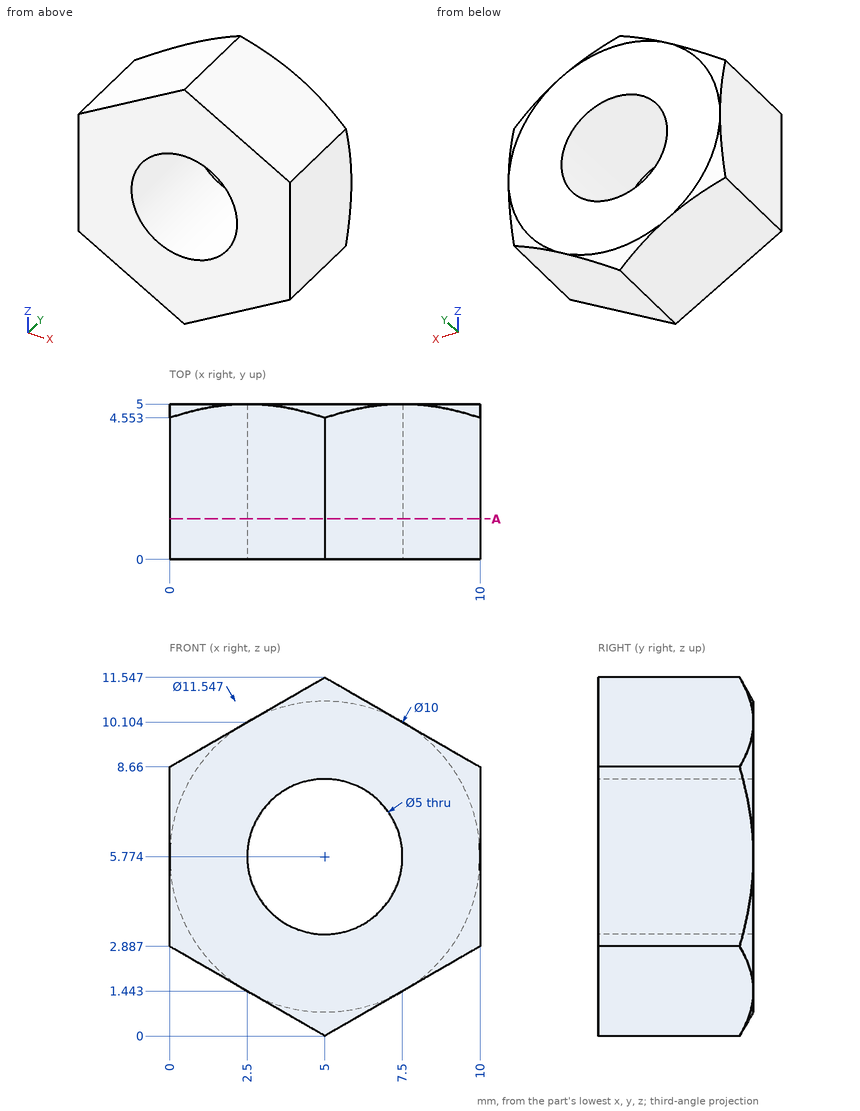
Study the drawing (mm; zero at the part's minimum x, y, z) and answer. Give positions to 0.01 mm unless a question says otherwise; leave off trailing zeros. Write each loop counter-clockwise with the first axis right and the second up, starting at its lowest first coordinate (ties: lowest second). Pieces come first, ordered by that corner, then holes. Notation, with made-up numbers: (-10.75, -27) - (37.25, -27) arc R22 ccw to (37.25, -9) - close; hole circle Ø10 at (52, 61.5). An arc over 180 degrees is marked (long way). One line per question, with ' | ' between items. Start each with the question number.
1. Straight lines are drawn through the part: line 1 (X direction, y = 2.4, z = 5.5) (1 decimal); line 2 (X direction, y = 3.55, z = 8) (1 decimal); line 3 (Z direction, x = 7, y = 4.05) (1 decimal). For each, find the intervals that lie inside material, in ascending order.
2. Given P1, Ø1, axis at y = 1.5, z = 1.5, coming from the +X side (1 decimal); P2, Ø1.5, axis at x = 1.5, y = 3, coming from the -Z side; P3, Ø2, axis at x = 7.5, y = 4, coming from the +Z side, each flat-ended and moving along its own axis, determine where each tip first touches the part or whether it passes through.
3. Section A-A, the plane y = 1.3 is taken. Determine the outline of the cut face in (x, z).
Result:
1) line 1: x = 0 to 2.5, 7.5 to 10 | line 2: x = 0 to 3.9, 6.1 to 10 | line 3: z = 1.2 to 4.3, 7.3 to 10.4
2) P1: stops at x = 8.5 | P2: stops at z = 1.59 | P3: stops at z = 10.68
3) outline: (0, 2.89) - (5, 0) - (10, 2.89) - (10, 8.66) - (5, 11.55) - (0, 8.66) - close; hole circle Ø5 at (5, 5.77)
